Verification items for this drawing (mm, ordinates from the low corner). A direction names the side the tool comes from. Round coordinates to 2 decimals unless told otherwise and drop trailing zeros. Loops run counter-clockwise (first coordinate to the right, second up) from the corner with the lowest first, then second, coordinate; pieces in that order, holes last. Notation, with made-up numbers: (87, 85.25) - (108, 85.25) arc R26 cw to (108, 122.25) - close; hole circle Ø8 at (-27, 40.5). An arc over 180 degrees is marked (long way). Answer in a Markdown table with one row per item. Add a question column.
(1) Mould release check, pull along Z, two halves, no side actions. Record for the marked faces 1, 2 and 3: +Z half, -Z half, draft (parallel to the pull), parting line (faces both ways), or undercut.
(2) Cross-section at A-A on y = 81. Enter the section's corners in (x, z) (1 decimal), then the cut area to 3 significant figures.
(3) Cross-section at C-C on x = 25. Enter the section's corners in (y, z).
(4) Cross-section at B-B on z = 83. Enter the section's corners in (x, y).
(5) Cross-section at D-D on z = 46. Enter the section's corners in (x, y).
(6) Gauge pin test, flat ends, axial feed: pin 1 (5 mm diameter, centred on y = 20.5, z = 71, fed in from +X); pin 2 (4 mm diameter, centred on x = 131, z = 73, fed in from +Y); pin 3 (1.5 mm diameter, centred on x = 30.5, y = 49, fed in from +Z). Record the tip position at first contact, or that the pin passes through.
(7) Access from +Z, -Z, +X, -X, +Y, -Y to the whole of each face (thin tool, end or side, straight path). Record for the marked faces 4, 5 and 6.
(8) Thickness scan on line 1 along X through (y, z) = (4, 20); line 2 along Z through (x, y) = (201.5, 6.5); line 3 along Y through (x, z) = (172.5, 67.5). Record the ranges inside material, lowest first.
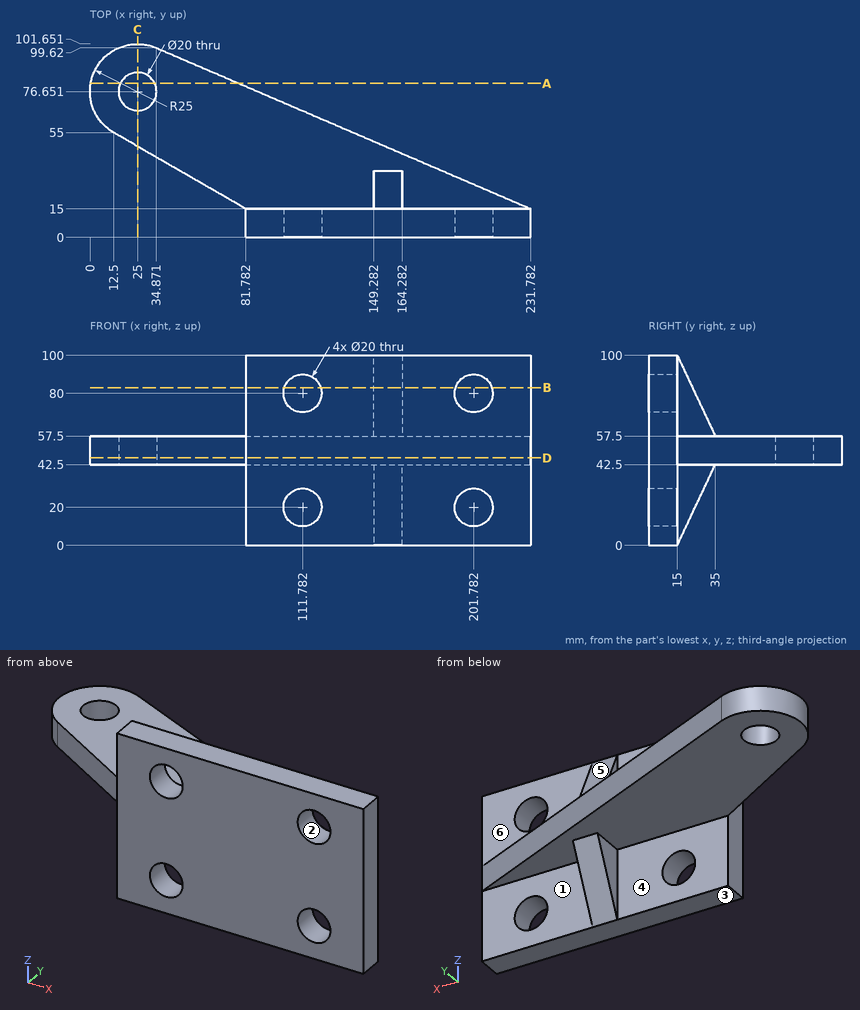
Answers:
| question | item | result |
|---|---|---|
| 1 | face 1 | draft |
| 1 | face 2 | undercut |
| 1 | face 3 | -Z half |
| 2 | outline | (0.4, 42.5) - (16, 42.5) - (16, 57.5) - (0.4, 57.5) - close; (34, 42.5) - (78.2, 42.5) - (78.2, 57.5) - (34, 57.5) - close |
| 2 | area | 897 mm^2 |
| 3 | outline | (47.78, 42.5) - (66.65, 42.5) - (66.65, 57.5) - (47.78, 57.5) - close; (86.65, 42.5) - (101.65, 42.5) - (101.65, 57.5) - (86.65, 57.5) - close |
| 4 | outline | (81.78, 0) - (102.24, 0) - (102.24, 15) - (81.78, 15) - close; (121.32, 0) - (192.24, 0) - (192.24, 15) - (164.28, 15) - (164.28, 23) - (149.28, 23) - (149.28, 15) - (121.32, 15) - close; (211.32, 0) - (231.78, 0) - (231.78, 15) - (211.32, 15) - close |
| 5 | outline | (12.5, 55) - (81.78, 15) - (81.78, 0) - (231.78, 0) - (231.78, 15) - (34.87, 99.62) arc R25 ccw to start; hole circle Ø20 at (25, 76.65) |
| 6 | pin 1 | stops at x = 164.28 |
| 6 | pin 2 | stops at y = 15 |
| 6 | pin 3 | stops at z = 57.5 |
| 7 | face 4 | -Z, -X, +Y |
| 7 | face 5 | +Z, +X, -X, +Y |
| 7 | face 6 | +Z, +X, +Y |
| 8 | line 1 | x = 81.78 to 101.78, 121.78 to 191.78, 211.78 to 231.78 |
| 8 | line 2 | z = 0 to 10, 30 to 70, 90 to 100 |
| 8 | line 3 | y = 0 to 15 |
